Input: part model. Units: mm. Frame: model coordinates. Face numbers are marked on the shaded views. A direction names the side the tool comes from. Give positions to 0.01 mm unless a question says otherwise; leave off trailing zeros. Write each loop counter-clockwise with the first axis right and the second up, starting at its lowest first coordinate (ties: lowest second). Pieces come first, ordered by that corner, then holes. Notation, with made-up numbers: (57.5, 50.25) - (65.5, 50.25) arc R23 ccw to (65.5, 65.25) - close; hole circle Ø4 at (5.25, 68). An arc over 180 degrees is marked (long way). Answer as CSV lines item,"result".
```python
from build123d import *

# Parameters (mm, degrees)
F1_DEPTH = 1
F3_D     = 4.7625
F4_W     = 57.15
F4_H     = 25.4
F5_DEPTH = 50.8
F6_W     = 44.45
F6_H     = 31.75
F7_DEPTH = 25.4


with BuildPart() as f1:
    # F0 (on Top) → F1 (new body)
    with BuildSketch(Plane.XY):
        with BuildLine():
            ThreePointArc((-28.575, 12.7), (-41.275, 0), (-28.575, -12.7))
            Line((-28.575, -12.7), (-28.575, 12.7))
        make_face()
        with BuildLine():
            Line((-28.575, 12.7), (-28.575, -12.7))
            ThreePointArc((-28.575, -12.7), (-19.594744, -8.980256), (-15.875, 0))
            ThreePointArc((-15.875, 0), (-19.594744, 8.980256), (-28.575, 12.7))
        make_face()
        with BuildLine():
            ThreePointArc((-15.875, 0), (-19.594744, -8.980256), (-28.575, -12.7))
            Line((-28.575, -12.7), (28.575, -12.7))
            ThreePointArc((28.575, -12.7), (15.875, 0), (28.575, 12.7))
            Line((28.575, 12.7), (-28.575, 12.7))
            ThreePointArc((-28.575, 12.7), (-19.594744, 8.980256), (-15.875, 0))
        make_face()
        with BuildLine():
            ThreePointArc((28.575, 12.7), (15.875, 0), (28.575, -12.7))
            Line((28.575, -12.7), (28.575, 12.7))
        make_face()
        with BuildLine():
            Line((28.575, 12.7), (28.575, -12.7))
            ThreePointArc((28.575, -12.7), (37.555256, -8.980256), (41.275, 0))
            ThreePointArc((41.275, 0), (37.555256, 8.980256), (28.575, 12.7))
        make_face()
    extrude(amount=F1_DEPTH)

    # F3 (through all)
    with Locations(Plane.XY.offset(1)):
        with Locations((-35.687, 0), (35.687, 0)):
            Hole(F3_D / 2)

    # F4 (on face) → F5 (join)
    with BuildSketch(Plane.XY.offset(1)):
        Rectangle(F4_W, F4_H)
    extrude(amount=F5_DEPTH)

    # F6 (on Front) → F7 (join, symmetric)
    with BuildSketch(Plane.XZ):
        with Locations((0, 26.4)):
            Rectangle(F6_W, F6_H)
    extrude(amount=F7_DEPTH, both=True)


solid = f1.part
```
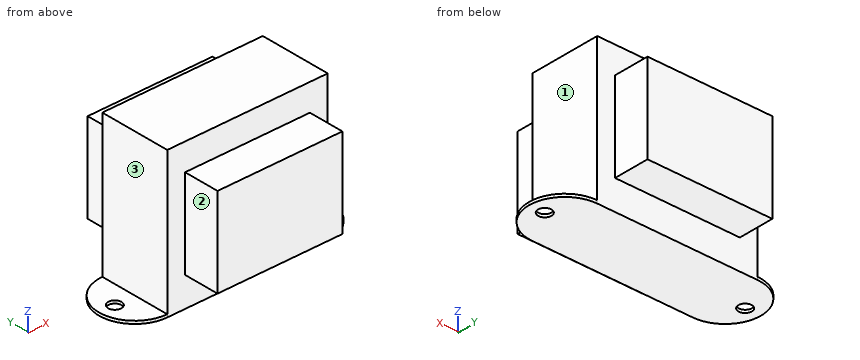
Item 1: Cut plane B-B on x = 5.5. Return the cut outline in (y, z) (3 decimals), plus the area to 3 significant figures.
The answers:
outline,"(-25.4, 10.525) - (-12.7, 10.525) - (-12.7, 0) - (12.7, 0) - (12.7, 10.525) - (25.4, 10.525) - (25.4, 42.275) - (12.7, 42.275) - (12.7, 51.8) - (-12.7, 51.8) - (-12.7, 42.275) - (-25.4, 42.275) - close"
area,"2,120 mm²"
Item 2: Cut plane A-A on z = 14. Return the cut outline in (x, y) (3 decimals).
The answers:
outline,"(-28.575, -12.7) - (-22.225, -12.7) - (-22.225, -25.4) - (22.225, -25.4) - (22.225, -12.7) - (28.575, -12.7) - (28.575, 12.7) - (22.225, 12.7) - (22.225, 25.4) - (-22.225, 25.4) - (-22.225, 12.7) - (-28.575, 12.7) - close"
Item 3: Contact query for flat-ended pins moving along their axis: pin 1 (10 mm diameter, centred on x = -33, y = 6, fed in from +Z); pin 2 (10 mm diameter, centred on x = 0.5, y = 19.5, fed in from -Z) (3 decimals); pin 3 (4 mm diameter, centred on y = -18.5, z = 31.5, fed in from +X) (3 decimals); pin 4 (1 mm diameter, centred on x = -7.5, y = -18.5, fed in from +Z) (3 decimals). Output: stop coordinate, or through.
The answers:
pin 1,"z = 51.8"
pin 2,"z = 10.525"
pin 3,"x = 22.225"
pin 4,"z = 42.275"
Item 4: Reachability of the marked faces 1, 2 and 3 from +Z, -Z, +X, -X, +Y, -Y: full face, straight path, thin tool, end or side. Return the list, or none.
The answers:
face 1,"+Z, +X, +Y, -Y"
face 2,"+Z, -Z, -X, -Y"
face 3,"+Z, -X, +Y, -Y"
Item 5: Cut plane D-D on y = 9. Return the cut outline in (x, z) (3 decimals).
The answers:
outline,"(-37.535, 0) - (37.535, 0) - (37.535, 1) - (28.575, 1) - (28.575, 51.8) - (-28.575, 51.8) - (-28.575, 1) - (-37.535, 1) - close"
Item 6: Ray query, line 1 (Z direction, x = 1, y = 14) (3 decimals); line 2 (X direction, y = 17, z = 33) (3 decimals); line 3 (Y direction, x = -25, z = 45). Return the intervals inside material, ascending. Write a range as from..to.
The answers:
line 1,"10.525..42.275"
line 2,"-22.225..22.225"
line 3,"-12.7..12.7"
Item 7: Cut plane C-C on x = 35.5. Return the cut outline in (y, z), plus the area to 3 significant figures.
The answers:
outline,"(-10.65, 0) - (-2.37, 0) - (-2.37, 1) - (-10.65, 1) - close; (2.37, 0) - (10.65, 0) - (10.65, 1) - (2.37, 1) - close"
area,"16.5 mm²"
